Part model, mm, in its own coordinate system. A direction names the side the tool comes from. Round coordinates to 2 decimals unless told otherwise and drop trailing zeros. Loops run counter-clockwise (first coordinate to the right, second up) from the corner with the lowest first, then second, coordinate; pieces in that order, holes last. Notation, with made-up numbers: (69.25, -37) - (106.25, -37) arc R15 ccw to (106.25, -25) - close; hole circle Ø5 at (84, -26.5). An arc over 180 degrees is marked (long way). Write each question's results on one line, items separated by ' | '. Start each with the question number.
(1) Cut at D-D, the plane x = 65.5. List the corners of the cut face in (y, z) (3 decimals).
(2) Cut at B-B, the plane y = -21. List the corners of the cut face in (x, z) (3 decimals), then the cut area to 3 significant figures.
(3) Flat gauge pins, fed straight in: P1, Ø1.5, axis at y = 40, z = 47, coming from the -X side; P2, Ø8, axis at x = -5.5, z = 33.5, coming from the +Y side; P3, Ø5, axis at y = 12.5, z = 22, coming from the -X side (3 decimals). Where does each tip first touch, or does it go through?
(4) Cut at A-A, the plane z = 7. List the corners of the cut face in (x, y) (3 decimals), then the cut area to 3 significant figures.
(5) Mould opens along X. For faces 1 (the face through (51, -14, 65.253)), 2 (the face through (39.464, 61.59, 0.133)), 3 (the face through (-41.275, -1, 0)), 4 (the face through (89.906, -0.91, 42.095)) say: released by +X, released by -X, zero draft, split by the parting line, or undercut.
(6) Cut at C-C, the plane y = 34. List the corners of the cut face in (x, z) (3 decimals), then the cut area to 3 significant figures.
(7) Tool access for faces 5 (the face through (44, -7.938, 64)), 6 (the face through (33, 25.4, 24)), 7 (the face through (33, -25.4, 24)), 8 (the face through (111.448, -19.457, 52.588)): list every direction of +Z, -Z, +X, -X, +Y, -Y with a clear straight run to the whole face (end or side of a thin tool).
(8) Drill centre lines: L1, parallel to Z at x = 32.5, y = -26 (3 decimals); L2, parallel to Z at x = 49.5, y = -25.5 (3 decimals); L3, parallel to Z at x = 11, y = -1 (3 decimals). Where is each one in solid material? Low to high.
from build123d import *

# Parameters (mm, degrees)
F1_DEPTH = 63.5
F0_W     = 25.4
F0_H     = 19.05
F2_DEPTH = 25.4
F3_DEPTH = 7.9375
F5_R     = 6.35


with BuildPart() as f1:
    # F0 (on Front) → F1 (new body, symmetric)
    with BuildSketch(Plane.XZ):
        Polygon((-41.275, -9.525), (41.275, -9.525), (41.275, 9.525), (22.225, 9.525), (-41.275, 9.525), align=None)
    extrude(amount=F1_DEPTH, both=True)

    # F0 (on Front) → F2 (join, symmetric)
    with BuildSketch(Plane.XZ):
        with BuildLine():
            Line((22.225, 9.525), (41.275, 9.525))
            Line((41.275, 9.525), (41.275, 30.3276))
            ThreePointArc((41.275, 30.3276), (45.9246798487, 41.5529201513), (57.15, 46.2026))
            Line((57.15, 46.2026), (64.5218447655, 46.2026))
            Line((64.5218447655, 46.2026), (64.5218447655, 65.2526))
            Line((64.5218447655, 65.2526), (57.15, 65.2526))
            ThreePointArc((57.15, 65.2526), (32.4542956671, 55.0233043329), (22.225, 30.3276))
            Line((22.225, 30.3276), (22.225, 9.525))
        make_face()
        with Locations((77.2218447655, 55.7276)):
            Rectangle(F0_W, F0_H)
    extrude(amount=F2_DEPTH, both=True)

    # F0 (on Front) → F3 (join, symmetric)
    with BuildSketch(Plane.XZ):
        with BuildLine():
            add(Edge.make_bspline(
                [(-41.275, 9.525), (-32.8745953739, 14.7935664281), (-3.6162044853, 80.2140161395), (57.15, 65.2526)],
                knots=[0, 0, 0, 0, 113.1063483044, 113.1063483044, 113.1063483044, 113.1063483044], degree=3))
            Line((-41.275, 9.525), (22.225, 9.525))
            Line((22.225, 9.525), (22.225, 30.3276))
            ThreePointArc((22.225, 30.3276), (32.4542956671, 55.0233043329), (57.15, 65.2526))
        make_face()
    extrude(amount=F3_DEPTH, both=True)

    # F0 (on Front) → F4 (revolve)
    with BuildSketch(Plane.XZ):
        Polygon((64.5218447655, 66.675), (64.5218447655, 65.2526), (89.9218447655, 65.2526), (89.9218447655, 46.2026), (89.9218447655, 38.1), (115.3218447655, 38.1), (115.3218447655, 66.675), align=None)
    revolve(axis=Axis((64.5218447655, 0, 52.3875), (0, 0, 1)))

    # F5
    f5_edges = [f1.edges().sort_by_distance(p)[0] for p in [
        (41.275, -63.5, 0),
        (-41.275, -63.5, 0),
        (41.275, 63.5, 0),
        (-41.275, 63.5, 0),
    ]]
    fillet(f5_edges, radius=F5_R)


solid = f1.part
A:
1) outline: (-50.791, 38.1) - (-25.381, 38.1) - (-25.381, 46.203) - (25.381, 46.203) - (25.381, 38.1) - (50.791, 38.1) - (50.791, 66.675) - (-50.791, 66.675) - close
2) outline: (-41.275, -9.525) - (41.275, -9.525) - (41.275, 30.328) arc R15.875 cw to (43.308, 38.1) - (50.233, 38.1) - (50.233, 44.617) arc R15.875 cw to (57.15, 46.203) - (78.81, 46.203) - (78.81, 38.1) - (110.778, 38.1) - (110.778, 66.675) - (18.266, 66.675) - (18.266, 38.1) - (23.101, 38.1) arc R34.925 ccw to (22.225, 30.328) - (22.225, 9.525) - (-41.275, 9.525) - close; hole (50.233, 64.561) arc R34.925 cw to (57.15, 65.253) - (50.233, 65.253) - close | area: 4,530 mm2
3) P1: x = 32.27 | P2: y = 7.94 | P3: x = 22.225
4) outline: (-41.275, -57.15) arc R6.35 ccw to (-34.925, -63.5) - (34.925, -63.5) arc R6.35 ccw to (41.275, -57.15) - (41.275, 57.15) arc R6.35 ccw to (34.925, 63.5) - (-34.925, 63.5) arc R6.35 ccw to (-41.275, 57.15) - close | area: 10,400 mm2
5) face 1: undercut | face 2: released by +X | face 3: released by -X | face 4: undercut
6) outline: (-41.275, -9.525) - (41.275, -9.525) - (41.275, 9.525) - (-41.275, 9.525) - close; (26.777, 38.1) - (102.266, 38.1) - (102.266, 66.675) - (26.777, 66.675) - close | area: 3,730 mm2
7) face 5: none | face 6: +X, -X, +Y | face 7: +X, -X, -Y | face 8: +Z
8) L1: -9.525 to 9.525, 38.1 to 66.675 | L2: 38.1 to 66.675 | L3: -9.525 to 60.962
